Geometry: see drawing. Coordinates: mm, zero at the bounding-box minimum. A direction names the side the tool comes from. Round coordinates to 2 decimals unless told otherwise and drop trailing zeros. Loops run counter-clockwise (first coordinate to the right, second up) from the corner with the lowest first, then second, coordinate; pieces in that order, holes last.
(1) First-contact query: pin 1 Ø1.8 at (x, z) = (17.5, 17.5) entering from +Y; pin 2 Ø1.5 at (y, z) = (2, 21) entering from +X; pin 3 Ø3.5 at (x, z) = (17.325, 17.325) entering from -Y. Flat tips, straight axial feed; report the tip coordinate or a pass-through.
(2) Section A-A, the plane z = 25. Return the cut outline in (x, y).
(3) Material intervals for probe 1 along X at (y, z) = (8.25, 17.5); probe 2 along Y at (x, z) = (5, 12.5); probe 3 along X at (y, z) = (3.5, 19.5), sorted ascending.
(4) Section B-B, the plane x = 16.5. Return the cut outline in (y, z).
(5) Section D-D, the plane z = 30.5. Return the cut outline in (x, y).
(6) Section C-C, the plane y = 5.5. Return the cut outline in (x, z) (3 decimals), plus the area to 3 significant figures.
(7) Mould query, pull axis Z, two halves, no side actions, for the marked faces 1, 2, 3 and 4. Classes: pulls with the +Z half, pulls with the -Z half, needs draft (parallel to the pull), parting line crosses it, or undercut.
(8) Set-up query: the marked faces 5, 6 and 7. Return all of +Z, -Z, +X, -X, +Y, -Y with unobstructed straight access to the full face (end or side cutting, diameter ignored); none if empty.
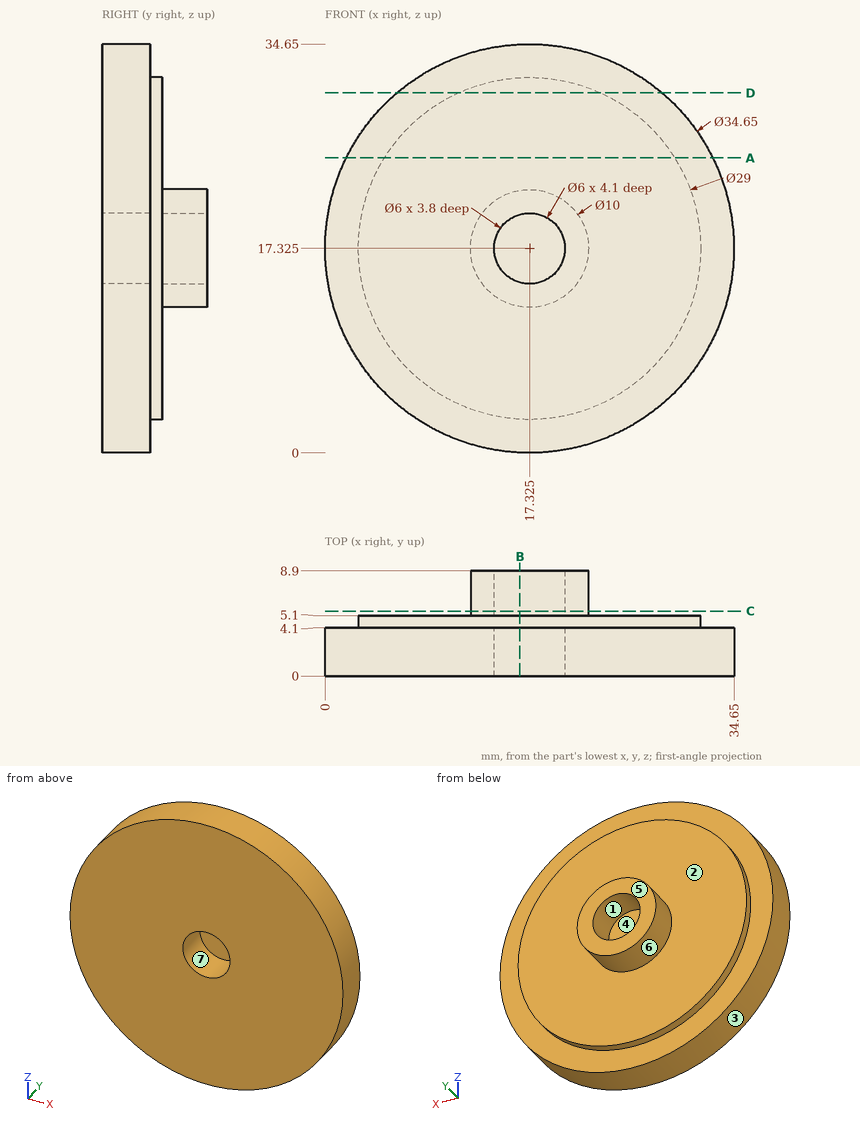
Output values:
1. pin 1: stops at y = 5.1
1. pin 2: stops at x = 34.4
1. pin 3: stops at y = 4.1
2. outline: (1.79, 0) - (32.86, 0) - (32.86, 4.1) - (29.63, 4.1) - (29.63, 5.1) - (5.02, 5.1) - (5.02, 4.1) - (1.79, 4.1) - close
3. probe 1: x = 12.33 to 14.33, 20.32 to 22.32
3. probe 2: y = 0 to 5.1
3. probe 3: x = 0.14 to 15.26, 19.39 to 34.51
4. outline: (0, 0.02) - (4.1, 0.02) - (4.1, 2.85) - (5.1, 2.85) - (5.1, 12.39) - (8.9, 12.39) - (8.9, 14.44) - (5.1, 14.44) - (5.1, 20.21) - (8.9, 20.21) - (8.9, 22.26) - (5.1, 22.26) - (5.1, 31.8) - (4.1, 31.8) - (4.1, 34.63) - (0, 34.63) - (0, 20.21) - (4.1, 20.21) - (4.1, 14.44) - (0, 14.44) - close
5. outline: (6.07, 0) - (28.58, 0) - (28.58, 4.1) - (23.38, 4.1) - (23.38, 5.1) - (11.27, 5.1) - (11.27, 4.1) - (6.07, 4.1) - close
6. outline: circle Ø10 at (17.325, 17.325); hole circle Ø6 at (17.325, 17.325)
6. area: 50.3 mm2
7. face 1: undercut
7. face 2: needs draft
7. face 3: parting line crosses it
7. face 4: undercut
8. face 5: +Z, -Z, +X, -X, +Y
8. face 6: +Y
8. face 7: -Y
